```python
from build123d import *

# Parameters (mm, degrees)
F1_DEPTH      = 15
F1_DEPTH_BACK = 15


with BuildPart() as f1:
    # F0 (on Front) → F1 (new body, two sides)
    with BuildSketch(Plane.XZ) as f1_sk:
        Polygon((0, 20), (0, 0), (-13, 0), (-16, 0), (-19, 0), (-19, 20), (-22, 20), (-22, 0), (-22, -12), (-16, -12), (-16, -32), (-13, -32), (-13, -29.301528), (-13, -12), (0, -12), (0, -32), (3, -32), (3, 20), align=None)
    extrude(amount=F1_DEPTH)
    extrude(f1_sk.sketch, amount=-F1_DEPTH_BACK)


solid = f1.part
```
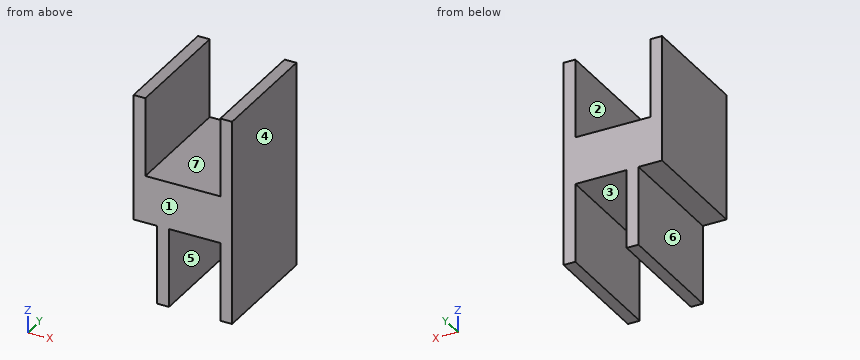
CAD build for the part. Positions are in the model's coordinates, mm. Face numbers are marked on the shaded views. A direction names the side the tool comes from. Round coordinates to 2 decimals unless told otherwise and drop trailing zeros. Write each loop counter-clockwise with the first axis right and the second up, starting at its lowest first coordinate (ties: lowest second). Pieces come first, ordered by that corner, then holes. Notation, with made-up numbers: (-30, 25.5) -> (13, 25.5) arc R19 ccw to (13, 30.5) -> close; hole circle Ø3 at (76, -5). An arc over 180 degrees is marked (long way). Answer in a Markdown table with one row per item. Add a question column.
Item 1: Saw through at A-A, the plane z = -26. Write the cut outline in (x, y).
Item 2: Drill centre lines: line 1 (X direction, y = -12, z = -29); line 2 (X direction, y = 7, z = 4); line 3 (Z direction, x = -16.25, y = 5.75). Where is each one in solid material? Low to high. Write a range as from..to.
Item 3: Saw through at C-C, the plane x = -4.75. Write the cut outline in (y, z).
Item 4: Drop flat-ended pins along their axis: pin 1 Ø1.5 at (x, y) = (-11, -8) entering from -Z; pin 2 Ø8 at (x, z) = (-11, 7) entering from +Y; pin 3 Ø6 at (y, z) = (1.5, -20.5) entering from -X. Give the stop position or say it passes through.
Item 5: Which spindle directions (+Z, -Z, +X, -X, +Y, -Y) get a long thin tool onto all of the face, cutting with end or side? Do the marked faces 5, 6 and 7. Say none if no direction does.
Item 6: Mould opens along X. For the marked faces 1, 2, 3 and 4 say: pulls with the +X half, pulls with the -X half, needs draft (parallel to the pull), parting line crosses it, or undercut.
Item 7: Saw through at B-B, the plane y = 10.5. Write the cut outline in (x, z), then the cut area to 3 significant figures.
Findings below:
| question | item | result |
|---|---|---|
| 1 | outline | (-16, -15) -> (-13, -15) -> (-13, 15) -> (-16, 15) -> close; (0, -15) -> (3, -15) -> (3, 15) -> (0, 15) -> close |
| 2 | line 1 | x = -16..-13, 0..3 |
| 2 | line 2 | x = -22..-19, 0..3 |
| 2 | line 3 | z = -12..0 |
| 3 | outline | (-15, -12) -> (15, -12) -> (15, 0) -> (-15, 0) -> close |
| 4 | pin 1 | stops at z = -12 |
| 4 | pin 2 | passes through |
| 4 | pin 3 | stops at x = -16 |
| 5 | face 5 | -Z, +Y, -Y |
| 5 | face 6 | -Z, -X, +Y, -Y |
| 5 | face 7 | +Z, +Y, -Y |
| 6 | face 1 | needs draft |
| 6 | face 2 | undercut |
| 6 | face 3 | undercut |
| 6 | face 4 | pulls with the +X half |
| 7 | outline | (-22, -12) -> (-16, -12) -> (-16, -32) -> (-13, -32) -> (-13, -12) -> (0, -12) -> (0, -32) -> (3, -32) -> (3, 20) -> (0, 20) -> (0, 0) -> (-19, 0) -> (-19, 20) -> (-22, 20) -> close |
| 7 | area | 540 mm^2 |
